Check sheet for the modelled part. Datum: model origin and axes. Units: mm. Face numbers are marked on the shaded views. A direction names the side the tool comes from. Give positions to 0.01 mm unless a question says otherwise; leave off trailing zeros. Order: outer loops, then holes, each group sorted by start corner. A loop starts at its lowest first (then second) coordinate and runs counter-clockwise, first axis right, second up. Notation, with made-up numbers: M -35,45.25 L 24,45.25 A19 ccw 24,65.25 Z; hole C 29.5,51.25 d10. An arc over 180 degrees is marked long. Answer in a Markdown table with one row per item. Add a question column.
from build123d import *

# Parameters (mm, degrees)
EXTRUDE_THIN1_DEPTH                       = 150
SKETCH2_OUTSIDE_W                         = 349.23
SKETCH2_OUTSIDE_H                         = 219.23
CUT_EXTRUDE1_DEPTH                        = 337.154726279
SKETCH3_R                                 = 30
CUT_EXTRUDE2_DEPTH                        = 323.116973634
CUT_EXTRUDE3_START                        = -15
CUT_EXTRUDE3_DEPTH                        = 10
SKETCH5_W                                 = 100
SKETCH5_H                                 = 2
CUT_EXTRUDE4_DEPTH                        = 323.116973634
CBORE_START                               = 14.1
CBORE_SLOT_FOR_M24_HEX_HEAD_BOLT1_DEPTH   = 15.9
CBORE_SLOT_FOR_M24_HEX_HEAD_BOLT1_2_DEPTH = 14.1
CBORE_FOR_M10_HEX_HEAD_BOLT1_D            = 11
CBORE_FOR_M10_HEX_HEAD_BOLT1_CBORE_D      = 21.48
CBORE_FOR_M10_HEX_HEAD_BOLT1_CBORE_DEPTH  = 6.85
CUT_EXTRUDE5_DEPTH                        = 303.31664336


# Read off the part's stored shape, not the designer's step: CBORE SLOT for M24 Hex Head Bolt1
with BuildPart() as part:
    # Sketch1 → Extrude-Thin1 (new body)
    with BuildSketch(Plane(origin=(0, 0, 0), x_dir=(1, 0, 0), z_dir=(0, 1, 0))):
        with BuildLine():
            Line((0, 0), (-96.684617092, 0))
            ThreePointArc((-96.684617092, 0), (-117.815530179, -4.684610648), (-134.986839248, -17.860619516))
            Line((-134.986839248, -17.860619516), (-181.133234795, -72.855752194))
            ThreePointArc((-181.133234795, -72.855752194), (-188.001758422, -78.126155741), (-196.454123657, -80))
            Line((-196.454123657, -80), (-280, -80))
            Line((-280, -80), (-280, -110))
            Line((-280, -110), (-196.454123657, -110))
            ThreePointArc((-196.454123657, -110), (-175.32321057, -105.315389352), (-158.151901501, -92.139380484))
            Line((-158.151901501, -92.139380484), (-112.005505955, -37.144247806))
            ThreePointArc((-112.005505955, -37.144247806), (-105.136982327, -31.873844259), (-96.684617092, -30))
            Line((-96.684617092, -30), (0, -30))
            Line((0, -30), (0, 0))
        make_face()
    extrude(amount=-EXTRUDE_THIN1_DEPTH)

    # Sketch2 outside → Cut-Extrude1 (cut, through all)
    with BuildSketch(Plane.XY):
        with Locations((-140, -75)):
            Rectangle(SKETCH2_OUTSIDE_W, SKETCH2_OUTSIDE_H)
        with BuildLine():
            Line((0, 0), (-234.676511429, -71.747809761))
            ThreePointArc((-234.676511429, -71.747809761), (-261.233833478, -121.694868189), (-211.286775051, -148.252190239))
            Line((-211.286775051, -148.252190239), (-95, -112.699755258))
            add(Edge.make_bspline(
                [(-95, -112.699755258), (-51.532544729, -99.410420536), (-36.95554526, -100), (0, -100)],
                knots=[0, 0, 0, 0, 1, 1, 1, 1], degree=3))
            Line((0, -100), (0, 0))
        make_face(mode=Mode.SUBTRACT)
    extrude(amount=CUT_EXTRUDE1_DEPTH, mode=Mode.SUBTRACT)

    # Sketch3 → Cut-Extrude2 (cut, through all)
    with BuildSketch(Plane.XY.offset(110)):
        with Locations(Location((-222.98164324, -110, 0), (0, 0, 27.840553026))):
            Circle(SKETCH3_R)
    extrude(amount=-CUT_EXTRUDE2_DEPTH, mode=Mode.SUBTRACT)

    # Sketch4 → Cut-Extrude3 (cut, symmetric)
    with BuildSketch(Plane.XY.offset(110).offset(CUT_EXTRUDE3_START)):
        with BuildLine():
            Line((-222.98164324, -68.172329741), (-222.98164324, -72.5))
            ThreePointArc((-222.98164324, -72.5), (-260.48164324, -110), (-222.98164324, -147.5))
            Line((-222.98164324, -147.5), (-222.98164324, -150))
            ThreePointArc((-222.98164324, -150), (-262.542277774, -115.912376445), (-234.676511429, -71.747809761))
            Line((-234.676511429, -71.747809761), (-222.98164324, -68.172329741))
        make_face()
    extrude(amount=CUT_EXTRUDE3_DEPTH, both=True, mode=Mode.SUBTRACT)

    # Sketch5 → Cut-Extrude4 (cut, through all)
    with BuildSketch(Plane.XY.offset(110)):
        with Locations((-272.98164324, -110)):
            Rectangle(SKETCH5_W, SKETCH5_H)
    extrude(amount=-CUT_EXTRUDE4_DEPTH, mode=Mode.SUBTRACT)

    # CBORE SLOT for M24 Hex Head Bolt1 outlin → CBORE SLOT for M24 Hex Head Bolt1 (cut)
    with BuildSketch(Plane.XY.offset(CBORE_START)):
        with BuildLine():
            Line((0, -47.715), (-47, -47.715))
            ThreePointArc((-47, -47.715), (-69.285, -70), (-47, -92.285))
            Line((-47, -92.285), (0, -92.285))
            Line((0, -92.285), (0, -47.715))
        make_face()
    extrude(amount=CBORE_SLOT_FOR_M24_HEX_HEAD_BOLT1_DEPTH, mode=Mode.SUBTRACT)

    # CBORE SLOT for M24 Hex Head Bolt1 2 outl → CBORE SLOT for M24 Hex Head Bolt1 2 (cut)
    with BuildSketch(Plane.XY):
        with BuildLine():
            Line((0, -83), (0, -57))
            Line((0, -57), (-47, -57))
            ThreePointArc((-47, -57), (-60, -70), (-47, -83))
            Line((-47, -83), (0, -83))
        make_face()
    extrude(amount=CBORE_SLOT_FOR_M24_HEX_HEAD_BOLT1_2_DEPTH, mode=Mode.SUBTRACT)

    # CBORE for M10 Hex Head Bolt1 (through all)
    with Locations(Plane.XY.offset(30)):
        with Locations((-50, -32)):
            CounterBoreHole(CBORE_FOR_M10_HEX_HEAD_BOLT1_D / 2, CBORE_FOR_M10_HEX_HEAD_BOLT1_CBORE_D / 2, CBORE_FOR_M10_HEX_HEAD_BOLT1_CBORE_DEPTH)

    # Sketch11 → Cut-Extrude5 (cut, through all)
    with BuildSketch(Plane(origin=(-47.437557366, 0, -39.80483689), x_dir=(0.6427876096865384, 0, -0.7660444431189788), z_dir=(0.7660444431189788, 0, 0.6427876096865384))):
        with BuildLine():
            Line((-159.78881321, -80.089014291), (-115.633379107, -71.411593064))
            ThreePointArc((-115.633379107, -71.411593064), (-106.827903218, -77.32459521), (-112.740905364, -86.130071099))
            Line((-112.740905364, -86.130071099), (-156.896339468, -94.807492326))
            ThreePointArc((-156.896339468, -94.807492326), (-165.701815356, -88.89449018), (-159.78881321, -80.089014291))
        make_face()
    extrude(amount=-CUT_EXTRUDE5_DEPTH, mode=Mode.SUBTRACT)


solid = part.part
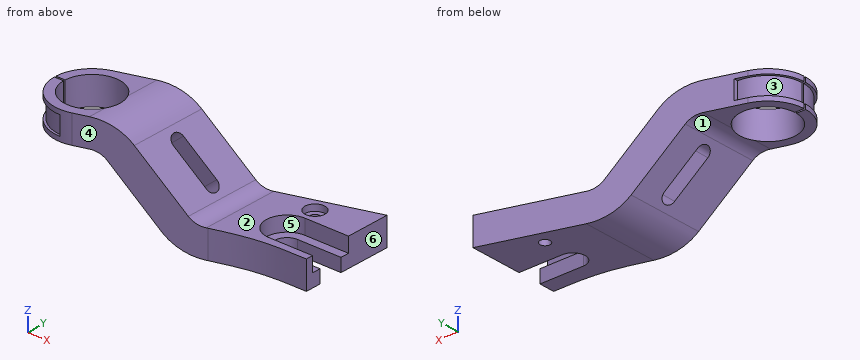
Q1. Go/stop test with flat-tipped pins: pin 1 (12 mm diameter, centred on x = -139, y = -102, fed in from -Z); pin 2 (2 mm diameter, centred on y = -70.5, z = 92.5, fed in from -X); pin 3 (19.5 mm diameter, centred on x = -250, y = -126, fed in from -Z); pin 4 (12 mm diameter, centred on x = -31.5, y = -81.5, fed in from -Z). Record where each tip stops, or that it passes through.
Q2. Cross-section at A-A (z = 58.5). Record the boundary of the cut face in (x, y), and give its area (3 significant figures).
Q3. Draft check along Y on the marked faces 3, 4, 5 and 6. Enter one of: pulls with the +Y half, pulls with the -Y half, needs draft (parallel to the pull), parting line crosses it, or undercut.
Q4. Cross-section at C-C (x = -247). Record the boundary of the cut face in (y, z).
Q5. Cross-section at B-B (y = -75.5). Record the boundary of the cut face in (x, z), and give its area (3 significant figures).
Q6. Thickness scan on probe 1 along X at (y, z) = (-135, 102); probe 2 along Y at (x, z) = (-20.5, 9.5); probe 3 along Y at (x, z) = (-128, 56). Record the ranges inside material, lowest first.
Q7. Tool access check on the marked faces 1 and 2. Record the directions out of +Z, -Z, +X, -X, +Y, -Y that give a thin tool (end or side, any length) a straight path to the whole face; none if there is none.
Q8. Cross-section at D-D (z = 101). Record the boundary of the cut face in (x, y), and give its area (3 significant figures).
Values follow:
| question | item | result |
|---|---|---|
| 1 | pin 1 | z = 15.63 |
| 1 | pin 2 | x = -222.98 |
| 1 | pin 3 | z = 80 |
| 1 | pin 4 | z = 0 |
| 2 | outline | M -169.09,-135.35 L -129.93,-123.38 L -129.93,-89.19 L -169.09,-94.14 Z; M -169.09,-78.85 L -129.93,-73.91 L -129.93,-39.72 L -169.09,-51.7 Z |
| 2 | area | 2,680 mm² |
| 3 | face 3 | pulls with the +Y half |
| 3 | face 4 | pulls with the -Y half |
| 3 | face 5 | undercut |
| 3 | face 6 | needs draft |
| 4 | outline | M -141.99,80 L -127.98,80 L -127.98,110 L -141.99,110 L -141.99,105 L -138.8,105 L -138.8,85 L -141.99,85 Z; M -92.02,80 L -78.01,80 L -78.01,85 L -81.2,85 L -81.2,105 L -78.01,105 L -78.01,110 L -92.02,110 Z |
| 5 | outline | M -243.22,80 L -196.45,80 A20 cw -181.13,72.86 L -158.12,45.43 L -135.14,64.71 L -158.15,92.14 A50 ccw -196.45,110 L -243.22,110 L -243.22,105 L -237.68,105 L -237.68,85 L -243.22,85 Z; M -139.48,23.21 L -134.99,17.86 A50 ccw -96.68,0 L -58.78,0 L -58.78,14.1 L -68.6,14.1 L -68.6,30 L -96.68,30 A20 cw -112.01,37.14 L -116.5,42.5 Z |
| 5 | area | 5,390 mm² |
| 6 | probe 1 | -250.93 to -239.56, -206.4 to -169.32 |
| 6 | probe 2 | -100.05 to -83, -57 to -6.27 |
| 6 | probe 3 | -122.79 to -88.57, -73.29 to -39.13 |
| 7 | face 1 | -Z, -X, +Y, -Y |
| 7 | face 2 | +Z, +X, +Y, -Y |
| 8 | outline | M -260.47,-111 A37.5 ccw -222.98,-147.5 L -222.98,-150 A40 ccw -211.29,-148.25 L -167.84,-134.97 L -167.84,-51.31 L -222.98,-68.17 L -222.98,-72.5 A37.5 ccw -260.47,-109 L -252.96,-109 A30 cw long -252.96,-111 Z |
| 8 | area | 3,970 mm² |
